from build123d import *

# Parameters (mm, degrees)
F0_R     = 1.905
F0_R_2   = 14.2875
F0_R_3   = 4.7625
F1_DEPTH = 12.7
F2_R     = 19.05
F3_DEPTH = 12.7
F5_DEPTH = 12.7
F6_R     = 1.905
F7_DEPTH = 12.7
F8_R     = 31.74999
F9_R     = 25.4
F10_R    = 12.7
F11_R    = 1.5875


# Not quite as in the source:
# - a fillet or chamfer is up to 0.001 mm smaller than in the source, because OpenCascade refuses the exact size


with BuildPart() as f1:
    # F0 (on Right) → F1 (new body)
    with BuildSketch(Plane.YZ):
        with BuildLine():
            Line((0, 355.6), (0, 0))
            Line((0, 0), (12.7, 0))
            ThreePointArc((12.7, 0), (50.8, 12.7), (88.9, 0))
            Line((88.9, 0), (431.8, 0))
            Line((431.8, 0), (431.8, 355.6))
            Line((431.8, 355.6), (0, 355.6))
        make_face()
        with Locations((57.329483813, 46.5276031344)):
            Circle(F0_R, mode=Mode.SUBTRACT)
        with Locations((143.6553005282, 86.7819925652)):
            Circle(F0_R, mode=Mode.SUBTRACT)
        with Locations((228.6, 63.5)):
            Circle(F0_R_2, mode=Mode.SUBTRACT)
        with Locations((330.2, 7.62)):
            Circle(F0_R_3, mode=Mode.SUBTRACT)
        with Locations((374.65, 63.5)):
            Circle(F0_R_2, mode=Mode.SUBTRACT)
        with Locations((133.35, 133.35)):
            Circle(F0_R_2, mode=Mode.SUBTRACT)
        with Locations((258.7563894819, 140.4545118063)):
            Circle(F0_R, mode=Mode.SUBTRACT)
    extrude(amount=F1_DEPTH)

    # F2 (on face) → F3 (cut, through all)
    with BuildSketch(Plane.YZ.offset(12.7)):
        with Locations((146.05, 23.05)):
            Circle(F2_R)
        with Locations((254, 23.05)):
            Circle(F2_R)
        with Locations((381, 23.0378)):
            Circle(F2_R)
        with Locations((200.025, 23.05)):
            Circle(F2_R)
    extrude(amount=-F3_DEPTH, mode=Mode.SUBTRACT)

    # F4 (on face) → F5 (cut, through all)
    with BuildSketch(Plane.YZ.offset(12.7)):
        Polygon((431.8, 355.6), (0, 355.6), (0, 279.4), (44.45, 279.4), (222.25, 279.4), (304.8, 238.125), (317.5, 101.6), (431.8, 101.6), (431.8, 247.65), align=None)
        with BuildLine():
            ThreePointArc((231.775, 158.5507812379), (146.2540591137, 234.1272060458), (44.45, 182.5368884968))
            ThreePointArc((44.45, 182.5368884968), (31.75, 133.35), (44.45, 84.1631115032))
            ThreePointArc((44.45, 84.1631115032), (50.9265271613, 73.9451927433), (58.5716384481, 64.5695039011))
            Line((58.5716384481, 64.5695039011), (113.1323420197, 101.0567142305))
            ThreePointArc((113.1323420197, 101.0567142305), (112.1703700265, 165.0207005635), (170.9171066227, 139.7))
            ThreePointArc((170.9171066227, 139.7), (171.3165429182, 136.5361605167), (171.45, 133.35))
            ThreePointArc((171.45, 133.35), (170.2668375807, 123.9289011764), (166.7908344859, 115.0929304409))
            Line((166.7908344859, 115.0929304409), (231.775, 158.5507812379))
        make_face()
    extrude(amount=-F5_DEPTH, mode=Mode.SUBTRACT)

    # F6 (on face) → F7 (cut, through all)
    with BuildSketch(Plane.YZ.offset(12.7)):
        with Locations((420.6875, 11.1125)):
            Circle(F6_R)
        with Locations((420.6875, 53.18125)):
            Circle(F6_R)
        with Locations((420.6875, 95.25)):
            Circle(F6_R)
        with Locations((298.45, 11.1125)):
            Circle(F6_R)
        with Locations((298.45, 95.25)):
            Circle(F6_R)
        with Locations((298.45, 53.18125)):
            Circle(F6_R)
        with Locations((11.1125, 23.8125)):
            Circle(F6_R)
        with Locations((122.05, 16.55)):
            Circle(F6_R)
        with Locations((170.05, 16.55)):
            Circle(F6_R)
        with Locations((230, 16.55)):
            Circle(F6_R)
        with Locations((278, 16.55)):
            Circle(F6_R)
        with Locations((357, 16.5378)):
            Circle(F6_R)
        with Locations((405, 16.5378)):
            Circle(F6_R)
        with Locations((11.1125, 273.05)):
            Circle(F6_R)
        with Locations((11.1125, 148.43125)):
            Circle(F6_R)
        with Locations((215.9725987291, 271.1144663844)):
            Circle(F6_R)
        with Locations((210.9129544728, 260.9951778719)):
            Circle(F6_R)
        with Locations((221.0322429853, 255.9355336156)):
            Circle(F6_R)
        with Locations((226.0918872416, 266.0548221281)):
            Circle(F6_R)
        with Locations((254, 124.079)):
            Circle(F6_R)
        with Locations((244.221, 114.3)):
            Circle(F6_R)
        with Locations((254, 104.521)):
            Circle(F6_R)
        with Locations((263.779, 114.3)):
            Circle(F6_R)
    extrude(amount=-F7_DEPTH, mode=Mode.SUBTRACT)

    # F8 (radius 31.75 in the source; OpenCascade refuses exactly that, so slightly less here)
    f8_edges = [f1.edges().sort_by_distance(p)[0] for p in [
        (6.35, 58.571638, 64.569504),
        (6.35, 113.132342, 101.056714),
        (6.35, 166.790834, 115.09293),
        (6.35, 231.775, 158.550781),
    ]]
    fillet(f8_edges, radius=F8_R)

    # F9
    f9_edges = [f1.edges().sort_by_distance(p)[0] for p in [
        (6.35, 222.25, 279.4),
    ]]
    fillet(f9_edges, radius=F9_R)

    # F10
    f10_edges = [f1.edges().sort_by_distance(p)[0] for p in [
        (6.35, 317.5, 101.6),
    ]]
    fillet(f10_edges, radius=F10_R)

    # F11
    f11_edges = [f1.edges().sort_by_distance(p)[0] for p in [
        (6.35, 431.8, 101.6),
        (6.35, 431.8, 0),
        (6.35, 0, 0),
        (6.35, 12.7, 0),
        (6.35, 88.9, 0),
        (6.35, 0, 279.4),
        (6.35, 304.8, 238.125),
    ]]
    fillet(f11_edges, radius=F11_R)


solid = f1.part
Could you check a few things on this model? Use its own coordinates, in mm. A direction names the side the tool comes from. Give positions to 0.01 mm unless a question says otherwise; leave off trailing zeros. Order: outer loops, then holes, each group sorted by start corner. A loop starts at its lowest first (then second) coordinate and runs counter-clockwise, first axis right, second up. Notation, with made-up numbers: (-36, -4) - (0, -4) arc R8 ccw to (0, 0) - close; hole circle Ø5 at (-15, 61.5). An arc over 180 degrees is marked (long way). One line per item, written item: value. Start each with the question number.
1. If I drill on probe 1 along Y at (x, z) = (3.5, 51); probe 2 along Z at (x, y) = (3.5, 405); probe 3 along Z at (x, y) = (2.75, 133.35), over which ranges is the centre line in solid material (lowest first)?
2. For P1, Ø3, axis at y = 230, z = 16.55, coming from the -X side, with a flat end and sliding along its axis, tell me the tip position at first contact or that it passes through.
3. For faces 1 (the face through (0, 165, 142)), 2 (the face through (6, 379, 101.6)), which set-ups out of +Z, -Z, +X, -X, +Y, -Y let a thin tool reach every point of the face, with its end or its side?
4. Thinking about a two-plate mould opening in Y: for faces 3 (the face through (6.26, 236.28, 75.55)), 4 (the face through (6.439, 310.574, 176.054)), 5 (the face through (6, 7, 0)), which applies, +Y half, -Y half, draft (parallel to the pull), parting line (faces both ways), or undercut?
5. Imagine slicing it at C-C on x = 10. Give the number of separate pieces and of enclosed holes in the cut face, plus the area to 3 significant figures.
6. Imagine slicing it at D-D on y = 312. List the corners of the cut face in (x, z) for me (3 decimals), plus the area to 3 significant figures.
7. Imagine slicing it at A-A on y = 133.35. List the corners of the cut face in (x, z) for me.
8. Imagine slicing it at B-B on z = 70.5. List the corners of the cut face in (x, y) for me, plus the area to 3 significant figures.
Values:
1. probe 1: 0 to 221.68, 235.52 to 367.73, 381.57 to 431.8
1. probe 2: 0 to 14.63, 18.44 to 101.6
1. probe 3: 0 to 8.85, 37.25 to 119.06, 147.64 to 171.45, 234.95 to 279.4
2. P1: through
3. face 1: +Z, -Z, -X, +Y, -Y
3. face 2: +Z, +X, -X, +Y
4. face 3: undercut
4. face 4: +Y half
4. face 5: draft
5. separate pieces: 1
5. enclosed holes: 35
5. area: 73,500 mm²
6. outline: (0, 0) - (12.7, 0) - (12.7, 160.725) - (0, 160.725) - close
6. area: 2,040 mm²
7. outline: (0, 0) - (12.7, 0) - (12.7, 8.85) - (0, 8.85) - close; (0, 37.25) - (12.7, 37.25) - (12.7, 119.06) - (0, 119.06) - close; (0, 147.64) - (12.7, 147.64) - (12.7, 171.45) - (0, 171.45) - close; (0, 234.95) - (12.7, 234.95) - (12.7, 279.4) - (0, 279.4) - close
8. outline: (0, 0) - (12.7, 0) - (12.7, 216.14) - (0, 216.14) - close; (0, 241.06) - (12.7, 241.06) - (12.7, 362.19) - (0, 362.19) - close; (0, 387.11) - (12.7, 387.11) - (12.7, 431.8) - (0, 431.8) - close
8. area: 4,850 mm²
